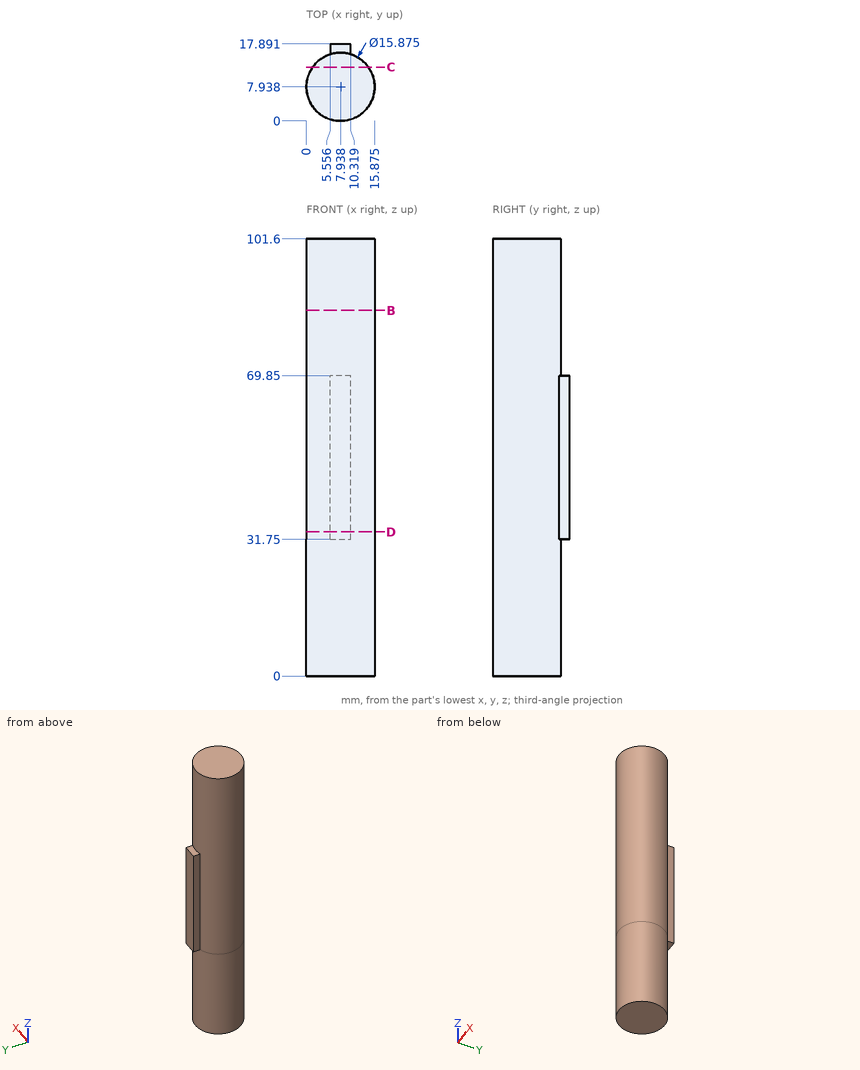
Input: dimensioned drawing with shaded views. Units: mm. Origin: part minimum x, y, z. Coordinates: 2 decimals unless noted, no trailing zeros. Order: outer loops, then holes, each group sorted by start corner. A loop starts at its lowest first (then second) coordinate and runs counter-clockwise, first axis right, second up.
Item 1: Material intervals for line 1 along Y through (x, z) = (7.75, 55.5); line 2 along X through (y, z) = (3.75, 64) (1 decimal); line 3 along X through (y, z) = (9, 24.5), sorted ascending.
Answer:
line 1: y = 0 to 17.89
line 2: x = 1.2 to 14.7
line 3: x = 0.07 to 15.8
Item 2: Contact query for flat-ended pins moving along their axis: P1, Ø6, axis at y = 15, z = 70, coming from the -X side; P2, Ø5, axis at x = 4.5, z = 87, coming from the -Y side (1 decimal); P3, Ø4, axis at y = 5, z = 33, coming from the +X side. Output: stop coordinate, or through.
Answer:
P1: stops at x = 1.12
P2: stops at y = 0.1
P3: stops at x = 15.82
Item 3: Section query C-C (y = 12.5). Output: boundary loops of the cut face in (x, z), then the cut area to 3 significant figures.
Answer:
outline: (1.44, 0) - (14.43, 0) - (14.43, 101.6) - (1.44, 101.6) - close
area: 1,320 mm2
Item 4: Section query B-B (z = 85). Output: boundary loops of the cut face in (x, y) (1 decimal).
Answer:
outline: circle Ø15.9 at (7.9, 7.9)
Item 5: Section query D-D (z = 33.5). Output: boundary loops of the cut face in (x, y) (1 decimal), then the cut area to 3 significant figures.
Answer:
outline: (5.6, 15.5) arc R7.9 ccw (long way) to (10.3, 15.5) - (10.3, 17.9) - (5.6, 17.9) - close
area: 208 mm2
